Design review of the part built by this model. Coordinates are the model's own, in mm. Face numbers are marked on the shaded views. A direction names the side the tool comes from. Coordinates: 2 decimals unless noted, no trailing zeros. Write each loop counter-clockwise with the first axis right and the second up, starting at its lowest first coordinate (ties: lowest second). Pieces come first, ordered by that corner, then holes.
Q1. Clearance check with flat-ended pins moving along their axes: pin 1 Ø12 at (x, y) = (-17, 1.5) entering from -Z; pin 2 Ø1.5 at (y, z) = (24.5, 29.5) entering from -X; pin 3 Ø12 at (x, y) = (-18, -10.5) entering from +Z; pin 4 Ø1.5 at (y, z) = (4.5, 10.5) entering from -X. State where each tip first meets the part, or that it passes through.
Q2. Add section B-B, the plane y = 10. Give the boundary of the cut face in (x, z), plus the area to 3 significant figures.
Q3. Add section A-A, the plane x = -38.1. Give the boundary of the cut face in (y, z).
Q4. Machinability: for the marked faces 1 and 2, which of the approach directions +Z, -Z, +X, -X, +Y, -Y give a long, thin tool a straight path to every point of the face, cutting with its end or side? Answer none if there is none.
Q5. To check wall thickness, follow probe 1 along X at (y, z) = (19.05, 2); probe 2 along Y at (x, z) = (-38.1, 2.2); probe 3 along Z at (x, y) = (-43, -6.5). State the ranges of each line that lie inside material, in increasing order.
Q6. Add section D-D, the plane z = 40.5. Give the boundary of the cut face in (x, y), plus the area to 3 significant figures.
Q7. Add section C-C, the plane x = -58.5. Give the boundary of the cut face in (y, z).
from build123d import *

# Parameters (mm, degrees)
F1_DEPTH = 31.75
F3_DEPTH = 25.4
F4_SIZE  = 0.3175


with BuildPart() as f1:
    # F0 (on Front) → F1 (new body, symmetric)
    with BuildSketch(Plane.XZ):
        with BuildLine():
            Line((-76.3057246804, 0), (-0.1057246804, 0))
            Line((-0.1057246804, 0), (-0.1057246804, 50.8))
            ThreePointArc((-0.1057246804, 50.8), (-4.595852741, 48.9401280605), (-6.4557246804, 44.45))
            Line((-6.4557246804, 44.45), (-6.4557246804, 12.7))
            ThreePointArc((-6.4557246804, 12.7), (-8.3155966199, 8.2098719395), (-12.8057246804, 6.35))
            Line((-12.8057246804, 6.35), (-69.9557246804, 6.35))
            ThreePointArc((-69.9557246804, 6.35), (-74.445852741, 4.4901280605), (-76.3057246804, 0))
        make_face()
    extrude(amount=F1_DEPTH, both=True)

    # F2 (on face) → F3 (cut)
    with BuildSketch(Plane(origin=(0, 0, 0), x_dir=(1, 0, 0), z_dir=(0, 0, -1))):
        with BuildLine():
            ThreePointArc((-34.925, -16.66875), (-42.06875, -19.05), (-34.925, -21.43125))
            Line((-34.925, -21.43125), (-34.925, -19.05))
            Line((-34.925, -19.05), (-34.925, -16.66875))
        make_face()
        with BuildLine():
            Line((-34.925, -19.05), (-34.925, -21.43125))
            ThreePointArc((-34.925, -21.43125), (-34.3349131609, -20.3050289464), (-34.13125, -19.05))
            ThreePointArc((-34.13125, -19.05), (-34.3349131609, -17.7949710536), (-34.925, -16.66875))
            Line((-34.925, -16.66875), (-34.925, -19.05))
        make_face()
    extrude(amount=-F3_DEPTH, mode=Mode.SUBTRACT)

    # F4
    f4_edges = [f1.edges().sort_by_distance(p)[0] for p in [
        (-41.275, 16.66875, 6.35),
        (-41.380725, 31.75, 6.35),
        (-41.380725, -31.75, 6.35),
        (-41.275, 16.66875, 0),
    ]]
    chamfer(f4_edges, length=F4_SIZE)


solid = f1.part
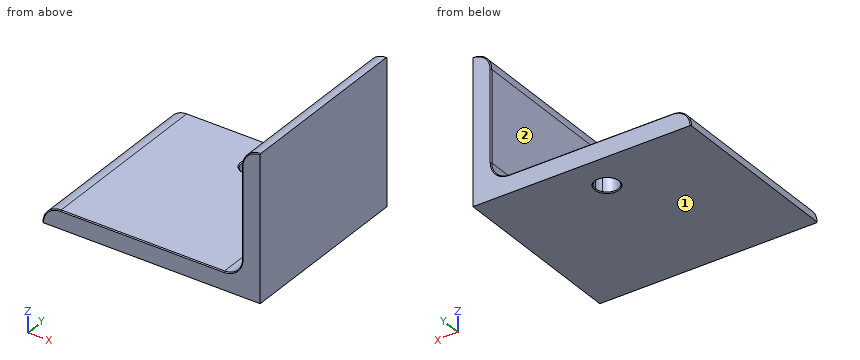
Here are the results:
1. pin 1: stops at z = 0
1. pin 2: stops at x = -6.46
1. pin 3: stops at z = 6.4
1. pin 4: stops at x = -7.18
2. outline: (-76.31, 0) - (-0.11, 0) - (-0.11, 50.8) arc R6.35 ccw to (-6.46, 44.45) - (-6.46, 12.7) arc R6.35 cw to (-12.81, 6.35) - (-69.96, 6.35) arc R6.35 ccw to start
2. area: 757 mm2
3. outline: (-31.75, 0) - (14.76, 0) - (15.08, 0.32) - (15.08, 6.03) - (14.76, 6.35) - (-31.43, 6.35) - (-31.75, 6.03) - close; (23.02, 0.32) - (23.34, 0) - (31.75, 0) - (31.75, 6.03) - (31.43, 6.35) - (23.34, 6.35) - (23.02, 6.03) - close
4. face 1: -Z, +X, -X, +Y, -Y
4. face 2: +Z, -X, +Y, -Y
5. probe 1: x = -75.98 to -42.07, -34.13 to -0.11
5. probe 2: y = -31.75 to 15.08, 23.02 to 31.75
5. probe 3: z = 0 to 6.35
6. outline: (-6.46, -31.43) - (-6.14, -31.75) - (-0.11, -31.75) - (-0.11, 31.75) - (-6.14, 31.75) - (-6.46, 31.43) - close
6. area: 403 mm2
7. outline: (-31.75, 0) - (31.75, 0) - (31.75, 6.03) - (31.43, 6.35) - (-31.43, 6.35) - (-31.75, 6.03) - close
